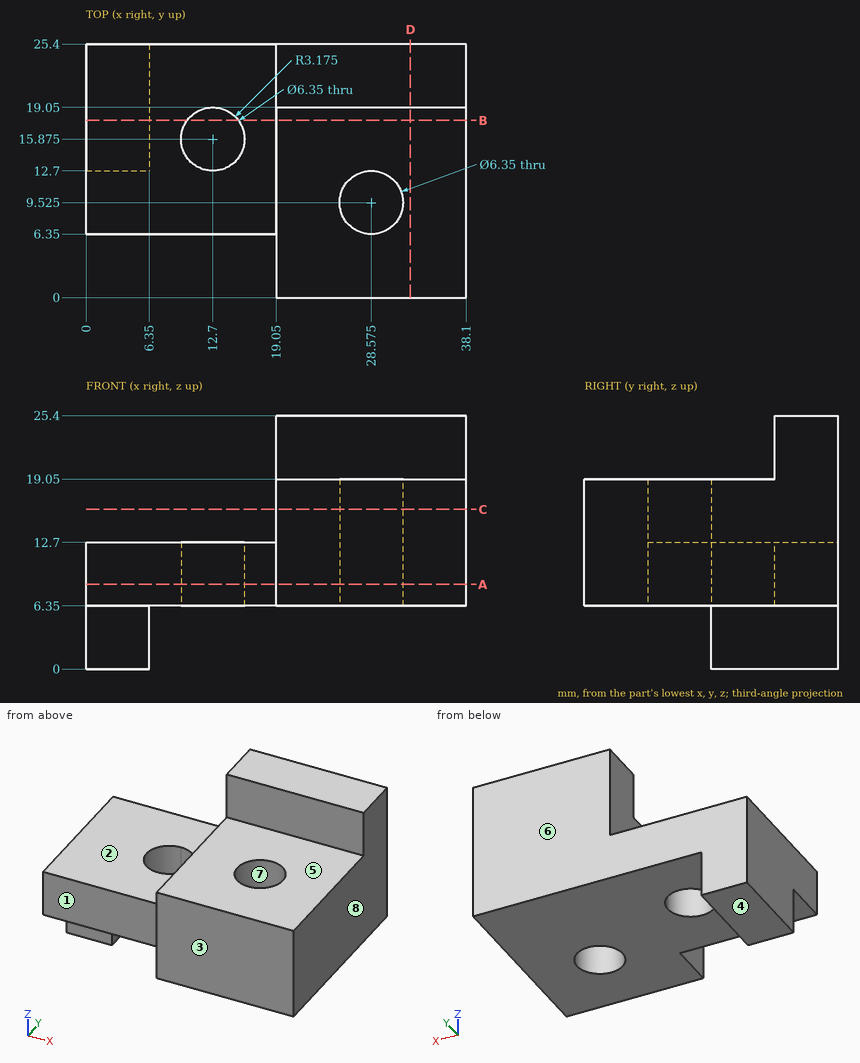
Here's the drawing with two shaded views (mm, measured from the low corner). I have some questions. A direction names the side the tool comes from. Coordinates: 2 decimals unless noted, no trailing zeros. Loops run counter-clockwise (first coordinate to the right, second up) from the corner with the lowest first, then second, coordinate; pieces in that order, holes last. Notation, with made-up numbers: (-3, 61) -> (37, 61) arc R21 ccw to (37, 72) -> close; hole circle Ø1 at (17, 67.5). An arc over 180 degrees is marked (long way). Answer in a Markdown table with one row per item.
(1) Will these pins go through, and if not, where does the flat tip stop? pin 1 Ø5.5 at (x, y) = (28.575, 9.525) entering from +Z; pin 2 Ø3 at (y, z) = (18.5, 4.5) entering from +X; pin 3 Ø10 at (x, y) = (12.7, 15.875) entering from -Z; pin 4 Ø2 at (y, z) = (6.5, 7) entering from -X.
Results found:
| item | result |
|---|---|
| pin 1 | passes through |
| pin 2 | stops at x = 6.35 |
| pin 3 | stops at z = 6.35 |
| pin 4 | stops at x = 0 |
(2) If I drill on probe 1 along X at (y, z) = (16.5, 13); probe 2 along X at (y, z) = (11, 16.5); probe 3 along Y at (x, z) = (12, 6.5), over which ranges is the centre line in solid material (lowest first)?
Results found:
| item | result |
|---|---|
| probe 1 | x = 19.05 to 38.1 |
| probe 2 | x = 19.05 to 25.76, 31.39 to 38.1 |
| probe 3 | y = 6.35 to 12.78, 18.97 to 25.4 |
(3) Imagine slicing it at A-A (z = 8.5). List the corners of the cut face in (x, y) for me (3 decimals).
Results found:
| item | result |
|---|---|
| outline | (0, 6.35) -> (19.05, 6.35) -> (19.05, 0) -> (38.1, 0) -> (38.1, 25.4) -> (0, 25.4) -> close; hole circle Ø6.35 at (12.7, 15.875); hole circle Ø6.35 at (28.575, 9.525) |
(4) For the marked faces 1, 2, 3, 4 and 5, which set-ups out of +Z, -Z, +X, -X, +Y, -Y let a thin tool reach every point of the face, with its end or its side?
Results found:
| item | result |
|---|---|
| face 1 | +Z, -Z, -X, -Y |
| face 2 | +Z, -X, +Y, -Y |
| face 3 | +Z, -Z, +X, -X, -Y |
| face 4 | -Z, +X, -X, +Y, -Y |
| face 5 | +Z, +X, -X, -Y |
(5) Imagine slicing it at C-C (z = 16). List the corners of the cut face in (x, y) for me (3 decimals), plus the area to 3 significant figures.
Results found:
| item | result |
|---|---|
| outline | (19.05, 0) -> (38.1, 0) -> (38.1, 25.4) -> (19.05, 25.4) -> close; hole circle Ø6.35 at (28.575, 9.525) |
| area | 452 mm^2 |
(6) Imagine slicing it at D-D (x = 32.5). List the corners of the cut face in (y, z) for me.
Results found:
| item | result |
|---|---|
| outline | (0, 6.35) -> (25.4, 6.35) -> (25.4, 25.4) -> (19.05, 25.4) -> (19.05, 19.05) -> (0, 19.05) -> close |
(7) Imagine slicing it at B-B (y = 17.75). List the corners of the cut face in (x, z) for me, plus the area to 3 significant figures.
Results found:
| item | result |
|---|---|
| outline | (0, 0) -> (6.35, 0) -> (6.35, 6.35) -> (10.14, 6.35) -> (10.14, 12.7) -> (0, 12.7) -> close; (15.26, 6.35) -> (38.1, 6.35) -> (38.1, 19.05) -> (19.05, 19.05) -> (19.05, 12.7) -> (15.26, 12.7) -> close |
| area | 371 mm^2 |
(8) Thinking about a two-plate mould opening in X: for the marked faces 6, 7 and 8, which applies, released by +X, released by -X, zero draft, split by the parting line, or undercut?
Results found:
| item | result |
|---|---|
| face 6 | zero draft |
| face 7 | undercut |
| face 8 | released by +X |
